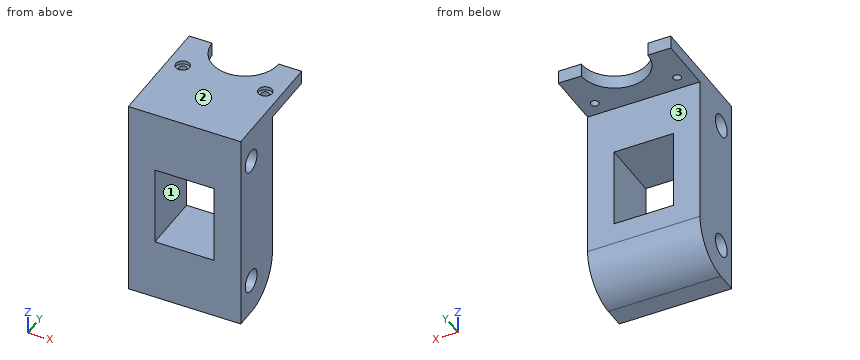
from build123d import *

# Parameters (mm, degrees)
SKETCH2_W                        = 42.3
SKETCH2_H                        = 76.2
BOSS_EXTRUDE1_DEPTH              = 15
SKETCH5_W                        = 42.3
SKETCH5_H                        = 42.3
MOUNTING_DEPTH                   = 5
SKETCH6_R                        = 12.5
SKETCH6_W                        = 42.3
SKETCH6_H                        = 21.15
PULLY_HOLE_DEPTH                 = 77.2
SKETCH8_R                        = 1.5
CUT_EXTRUDE_M3_DEPTH             = 77.2
SKETCH9_R                        = 2.58
SCREW_TOPS_DEPTH                 = 1.27
SKETCH11_W                       = 22.3
SKETCH11_H                       = 30
CUT_EXTRUDE1_DEPTH               = 37.15
SKETCH12_W                       = 42.3
SKETCH12_H                       = 76.2
SKETCH12_W_2                     = 22.3
SKETCH12_H_2                     = 30
F_7_85_CORRECTION_TO_MATCH_DEPTH = 7.85
SKETCH13_R                       = 4.25
CUT_EXTRUDE2_DEPTH               = 43.3
FILLET1_R                        = 15


with BuildPart() as part:
    # Sketch2 → Boss-Extrude1 (new body)
    with BuildSketch(Plane(origin=(0, 0, 0), x_dir=(1, 0, 0), z_dir=(0, 1, 0))):
        with Locations((1.968506494, -27.937012987)):
            Rectangle(SKETCH2_W, SKETCH2_H)
    extrude(amount=BOSS_EXTRUDE1_DEPTH)

    # Sketch5 → Mounting (add)
    with BuildSketch(Plane.XY.offset(66.037012987)):
        with Locations((1.968506494, 36.15)):
            Rectangle(SKETCH5_W, SKETCH5_H)
    extrude(amount=-MOUNTING_DEPTH)

    # Sketch6 → Pully Hole (cut, through all)
    with BuildSketch(Plane.XY.offset(66.037012987)):
        with Locations((1.968506494, 36.15)):
            Circle(SKETCH6_R)
        with Locations((1.968506494, 46.725)):
            Rectangle(SKETCH6_W, SKETCH6_H)
    extrude(amount=-PULLY_HOLE_DEPTH, mode=Mode.SUBTRACT)

    # Sketch8 → Cut-Extrude M3 (cut, through all)
    with BuildSketch(Plane.XY.offset(66.037012987)):
        with Locations((-13.531493506, 20.65)):
            Circle(SKETCH8_R)
        with Locations((17.468506494, 20.65)):
            Circle(SKETCH8_R)
    extrude(amount=-CUT_EXTRUDE_M3_DEPTH, mode=Mode.SUBTRACT)

    # Sketch9 → Screw Tops (cut)
    with BuildSketch(Plane.XY.offset(66.037012987)):
        with Locations((-13.531493506, 20.65)):
            Circle(SKETCH9_R)
        with Locations((17.468506494, 20.65)):
            Circle(SKETCH9_R)
    extrude(amount=-SCREW_TOPS_DEPTH, mode=Mode.SUBTRACT)

    # Sketch11 → Cut-Extrude1 (cut, through all)
    with BuildSketch(Plane.XZ):
        with Locations((1.968506494, 27.937012987)):
            Rectangle(SKETCH11_W, SKETCH11_H)
    extrude(amount=-CUT_EXTRUDE1_DEPTH, mode=Mode.SUBTRACT)

    # Sketch12 → 7.85 correction to match (add)
    with BuildSketch(Plane.XZ):
        with Locations((1.968506494, 27.937012987)):
            Rectangle(SKETCH12_W, SKETCH12_H)
        with Locations((1.968506494, 27.937012987)):
            Rectangle(SKETCH12_W_2, SKETCH12_H_2, mode=Mode.SUBTRACT)
    extrude(amount=F_7_85_CORRECTION_TO_MATCH_DEPTH)

    # Sketch13 → Cut-Extrude2 (cut, through all)
    with BuildSketch(Plane(origin=(23.118506494, 0, 0), x_dir=(0, 0, -1), z_dir=(1, 0, 0))):
        with Locations((-52.937012987, -0.35)):
            Circle(SKETCH13_R)
        with Locations((-2.937012987, -0.35)):
            Circle(SKETCH13_R)
    extrude(amount=-CUT_EXTRUDE2_DEPTH, mode=Mode.SUBTRACT)

    # Fillet1
    fillet1_edges = [part.edges().sort_by_distance(p)[0] for p in [
        (1.968506494, 15, -10.162987013),
    ]]
    fillet(fillet1_edges, radius=FILLET1_R)


solid = part.part
Input: part model. Units: mm. Frame: model coordinates. Face numbers are marked on the shaded views. A direction names the side the tool comes from. Round coordinates to 2 decimals unless told otherwise and drop trailing zeros. Write each loop counter-clockwise with the first axis right and the second up, starting at its lowest first coordinate (ties: lowest second). Pieces come first, ordered by that corner, then holes.
1) Reachability of the marked faces 1, 2 and 3 from +Z, -Z, +X, -X, +Y, -Y: full face, straight path, thin tool, end or side. Return the list, or none.
2) Cut plane C-C (y = 20.65). Return the cut outline in (x, z).
3) Contact query for flat-ended pins moving along their axis: P1, Ø24.5, axis at x = 0.5, y = 3.5, coming from the -Z side; P2, Ø4, axis at x = 17.47, y = 20.65, coming from the -Z side; P3, Ø1.5, axis at x = 18.5, y = 20, coming from the +Z side; P4, Ø21, axis at x = 2.5, z = 45.5, coming from the +Y side. Output: stop coordinate, or through.
4) Cut plane D-D (x = -2.5). Return the cut outline in (y, z).
5) Ray query, L1, parallel to Z at x = -2.5, y = 8; L2, parallel to X at y = 20, z = 62; L3, parallel to Y at x = 14.5, z = 12.5. Return the intervals inside material, ascending.
6) Cut plane A-A (z = 34). Return the cut outline in (x, y), then the cut area to 3 significant figures.
7) Cut plane B-B (x = 2.5). Return the cut outline in (y, z), then the cut area to 3 significant figures.
Geometry says:
1. face 1: +Y, -Y
1. face 2: +Z, +X, -X, +Y, -Y
1. face 3: -Z, +X, -X, +Y
2. outline: (-19.18, 61.04) - (-15.03, 61.04) - (-15.03, 64.77) - (-16.11, 64.77) - (-16.11, 66.04) - (-19.18, 66.04) - close; (-12.03, 61.04) - (15.97, 61.04) - (15.97, 64.77) - (14.89, 64.77) - (14.89, 66.04) - (-10.95, 66.04) - (-10.95, 64.77) - (-12.03, 64.77) - close; (18.97, 61.04) - (23.12, 61.04) - (23.12, 66.04) - (20.05, 66.04) - (20.05, 64.77) - (18.97, 64.77) - close
3. P1: stops at z = -10.16
3. P2: stops at z = 61.04
3. P3: stops at z = 64.77
3. P4: stops at y = 15
4. outline: (-7.85, -10.16) - (0, -10.16) arc R15 ccw to (15, 4.84) - (15, 12.94) - (-7.85, 12.94) - close; (-7.85, 42.94) - (15, 42.94) - (15, 61.04) - (24.48, 61.04) - (24.48, 66.04) - (-7.85, 66.04) - close; hole circle Ø8.5 at (-0.35, 2.94); hole circle Ø8.5 at (-0.35, 52.94)
5. L1: z = -7.85 to 12.94, 42.94 to 66.04
5. L2: x = -19.18 to -14.88, -12.18 to 16.12, 18.82 to 23.12
5. L3: y = -7.85 to 15
6. outline: (-19.18, -7.85) - (-9.18, -7.85) - (-9.18, 15) - (-19.18, 15) - close; (13.12, -7.85) - (23.12, -7.85) - (23.12, 15) - (13.12, 15) - close
6. area: 457 mm2
7. outline: (-7.85, -10.16) - (0, -10.16) arc R15 ccw to (15, 4.84) - (15, 12.94) - (-7.85, 12.94) - close; (-7.85, 42.94) - (15, 42.94) - (15, 61.04) - (23.66, 61.04) - (23.66, 66.04) - (-7.85, 66.04) - close; hole circle Ø8.5 at (-0.35, 2.94); hole circle Ø8.5 at (-0.35, 52.94)
7. area: 937 mm2
